Check sheet for the modelled part. Datum: model origin and axes. Units: mm. A direction names the side the tool comes from. Coordinates: 2 decimals unless noted, no trailing zeros. Loops run counter-clockwise (first coordinate to the right, second up) from the corner with the lowest first, then second, coordinate; pieces in that order, holes last. Notation, with made-up numbers: (-37, 25.25) -> (19, 25.25) arc R29 cw to (19, 45.25) -> close; hole circle Ø1 at (59.5, 17.5). An arc over 180 degrees is marked (long way). Use CSV: the item, a comma, the result in double quotes.
```python
from build123d import *

# Parameters (mm, degrees)
F0_W     = 50.8
F0_H     = 38.1
F1_DEPTH = 12.7
F2_W     = 50.8
F2_H     = 12.7
F3_DEPTH = 63.5
F4_W     = 12.7
F4_H     = 12.7
F5_DEPTH = 12.701
F6_R     = 12.7
F7_DEPTH = 12.701
F8_R     = 25.39999


# Not quite as in the source:
# - a fillet or chamfer is up to 0.001 mm smaller than in the source, because OpenCascade refuses the exact size


with BuildPart() as f1:
    # F0 (on Top) → F1 (new body)
    with BuildSketch(Plane.XY):
        with Locations((-25.4, 19.05)):
            Rectangle(F0_W, F0_H)
    extrude(amount=F1_DEPTH)

    # F2 (on face) → F3 (join)
    with BuildSketch(Plane(origin=(0, 0, 0), x_dir=(1, 0, 0), z_dir=(0, 0, -1))):
        with Locations((-25.4, -6.35)):
            Rectangle(F2_W, F2_H)
    extrude(amount=-F3_DEPTH)

    # F4 (on face) → F5 (cut, through all)
    with BuildSketch(Plane.XY.offset(12.7)):
        with Locations((-44.45, 31.75)):
            Rectangle(F4_W, F4_H)
    extrude(amount=-F5_DEPTH, mode=Mode.SUBTRACT)

    # F6 (on face) → F7 (cut, through all)
    with BuildSketch(Plane(origin=(0, 12.7, 0), x_dir=(-1, 0, 0), z_dir=(0, 1, 0))):
        with Locations((25.4, 38.1)):
            Circle(F6_R)
    extrude(amount=-F7_DEPTH, mode=Mode.SUBTRACT)

    # F8 (radius 25.4 in the source; OpenCascade refuses exactly that, so slightly less here)
    f8_edges = [f1.edges().sort_by_distance(p)[0] for p in [
        (-50.8, 6.35, 63.5),
        (0, 6.35, 63.5),
    ]]
    fillet(f8_edges, radius=F8_R)


solid = f1.part
```
1) Cross-section at D-D on y = 28. Record the boundary of the cut face in (x, z).
Answer below:
outline,"(-38.1, 0) -> (0, 0) -> (0, 12.7) -> (-38.1, 12.7) -> close"
2) Cross-section at C-C on z = 31.5. Record the boundary of the cut face in (x, y).
Answer below:
outline,"(-50.8, 0) -> (-36.25, 0) -> (-36.25, 12.7) -> (-50.8, 12.7) -> close; (-14.55, 0) -> (0, 0) -> (0, 12.7) -> (-14.55, 12.7) -> close"
3) Cross-section at B-B on x = -35. Record the boundary of the cut face in (y, z), and give its area (3 significant figures).
Answer below:
outline,"(0, 0) -> (38.1, 0) -> (38.1, 12.7) -> (12.7, 12.7) -> (12.7, 29.79) -> (0, 29.79) -> close; (0, 46.41) -> (12.7, 46.41) -> (12.7, 61.62) -> (0, 61.62) -> close"
area,"894 mm²"
4) Access from +Z, -Z, +X, -X, +Y, -Y to the whole of each face (thin tool, end or side, straight path). Record for faces 1 (the flat face through (-19, 38.1, 6)), 2 (the flat face through (-45, 25.4, 6)), 3 (the flat face through (-20, 12.7, 26)).
Answer below:
face 1,"+Z, -Z, +X, -X, +Y"
face 2,"+Z, -Z, -X, +Y"
face 3,"+Z, +X, -X, +Y"
5) Thickness scan on line 1 along Z through (x, y) = (-25.4, 5); line 2 along Z through (x, y) = (-16, 18.5); line 3 along X through (y, z) = (7, 38). Record the ranges inside material, lowest first. Write a range as from..to.
Answer below:
line 1,"z = 0..25.4, 50.8..63.5"
line 2,"z = 0..12.7"
line 3,"x = -50.8..-38.1, -12.7..0"
6) Go/stop test with flat-tipped pins: pin 1 Ø3 at (x, y) = (-28, 16.5) entering from +Z; pin 2 Ø4 at (y, z) = (35, 5.5) entering from -X; pin 3 Ø10 at (x, z) = (-13, 42) entering from -Y; pin 4 Ø10 at (x, z) = (-34, 22) entering from +Y. Record where each tip stops, or that it passes through.
Answer below:
pin 1,"stops at z = 12.7"
pin 2,"stops at x = -38.1"
pin 3,"stops at y = 0"
pin 4,"stops at y = 12.7"
